Here's how the part is built. I have some questions about the finished solid (model axes, mm). Give positions to 0.01 mm unless a question says otherwise; leave off trailing zeros. Loops run counter-clockwise (first coordinate to the right, second up) from the corner with the lowest first, then second, coordinate; pieces in that order, holes last. Notation, with made-up numbers: (16, 61) -> (45, 61) arc R32 ccw to (45, 90) -> close; hole circle Ø11 at (-6.75, -35). An arc over 180 degrees is marked (long way). Answer in a Markdown table with one row per item. Add a question column.
Item 1: If I drill on line 1 (Y direction, x = -1.5, z = 4.25); line 2 (X direction, y = 38.5, z = -1.75); line 3 (X direction, y = 84, z = -0.25), over which ranges is the centre line in solid material (lowest first)?
Item 2: For P1, Ø2, axis at x = 3, y = 10.5, coming from the -Z side; P2, Ø1.5, axis at y = 85, z = 1, coming from the +X side; P3, Ø1.5, axis at x = -3.5, y = 71.5, coming from the -Z side, each with a flat end and sliding along its axis, tell me the tip position at first contact or that it passes through.
Item 3: If we section it at A-A (y = 60): Write out the boundary of the cut face in (x, z), then the cut area to 3 significant figures.
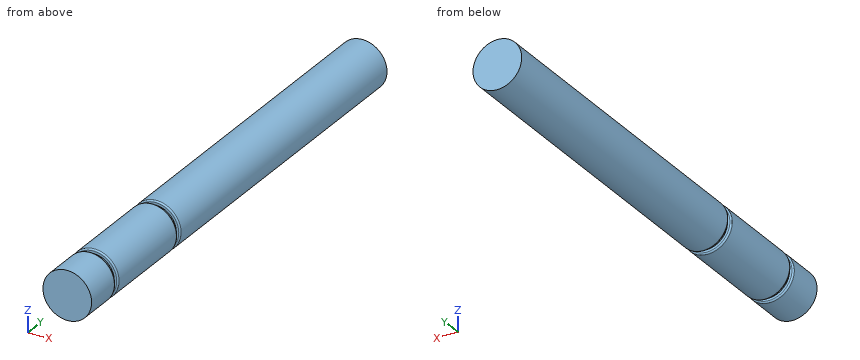
```python
from build123d import *

# Parameters (mm, degrees)
SKETCH1_R           = 5
BOSS_EXTRUDE1_DEPTH = 100
CUT_EXTRUDE1_START  = 30
SKETCH2_R           = 5
SKETCH2_R_2         = 4.2
CUT_EXTRUDE1_DEPTH  = 1
FILLET1_R           = 0.3
CUT_EXTRUDE2_START  = 8
SKETCH2_2_R         = 5
SKETCH2_2_R_2       = 4.2
CUT_EXTRUDE2_DEPTH  = 1
FILLET2_R           = 0.3


with BuildPart() as part:
    # Sketch1 → Boss-Extrude1 (new body)
    with BuildSketch(Plane(origin=(0, 0, 0), x_dir=(1, 0, 0), z_dir=(0, 1, 0))):
        Circle(SKETCH1_R)
    extrude(amount=BOSS_EXTRUDE1_DEPTH)

    # Sketch2 → Cut-Extrude1 (cut)
    with BuildSketch(Plane(origin=(0, 0, 0), x_dir=(1, 0, 0), z_dir=(0, 1, 0)).offset(CUT_EXTRUDE1_START)):
        Circle(SKETCH2_R)
        Circle(SKETCH2_R_2, mode=Mode.SUBTRACT)
    extrude(amount=-CUT_EXTRUDE1_DEPTH, mode=Mode.SUBTRACT)

    # Fillet1
    fillet1_edges = [part.edges().sort_by_distance(p)[0] for p in [
        (-5, 29, 0),
        (-5, 30, 0),
    ]]
    fillet(fillet1_edges, radius=FILLET1_R)

    # Sketch2_2 → Cut-Extrude2 (cut)
    with BuildSketch(Plane(origin=(0, 0, 0), x_dir=(1, 0, 0), z_dir=(0, 1, 0)).offset(CUT_EXTRUDE2_START)):
        Circle(SKETCH2_2_R)
        Circle(SKETCH2_2_R_2, mode=Mode.SUBTRACT)
    extrude(amount=CUT_EXTRUDE2_DEPTH, mode=Mode.SUBTRACT)

    # Fillet2
    fillet2_edges = [part.edges().sort_by_distance(p)[0] for p in [
        (-5, 9, 0),
        (-5, 8, 0),
    ]]
    fillet(fillet2_edges, radius=FILLET2_R)


solid = part.part
```
Recorded:
| question | item | result |
|---|---|---|
| 1 | line 1 | y = 0 to 8, 9 to 29, 30 to 100 |
| 1 | line 2 | x = -4.68 to 4.68 |
| 1 | line 3 | x = -4.99 to 4.99 |
| 2 | P1 | stops at z = -4.58 |
| 2 | P2 | stops at x = 4.99 |
| 2 | P3 | stops at z = -4.18 |
| 3 | outline | circle Ø10 at (0, 0) |
| 3 | area | 78.5 mm^2 |
